Here's the drawing with two shaded views (mm, measured from the low corner). I have some questions. A direction names the side the tool comes from. Round coordinates to 2 decimals unless told otherwise and drop trailing zeros. Order: outer loops, then holes, each group sorted by start corner. A loop starts at its lowest first (then second) coordinate and runs counter-clockwise, first axis right, second up.
Q1. If we section it at A-A (y = 8.5): Please give me the cut outline in (x, z), plus the area to 3 significant figures.
Q2. If we section it at D-D (z = 8): Please give me the cut outline in (x, y), plus the area to 3 significant figures.
Q3. For the marked faces 1 and 2, which set-ups out of +Z, -Z, +X, -X, +Y, -Y let a thin tool reach every point of the face, with its end or its side?
Q4. If I drill on line 1 (Z direction, x = 7.25, y = 3.5); line 2 (Y direction, x = 8.25, z = 32); line 3 (Y direction, x = 12.5, z = 44.5), over which ranges is the centre line in solid material (lowest first)?
Q5. Will these pins go through, and if not, where does the flat tip stop? P1, Ø8, axis at x = 3, z = 16.5, coming from the +Y side; P2, Ø2, axis at x = 14.5, z = 32, coming from the -Y side; P3, Ø2, axis at y = 2, z = 37, coming from the +X side.
Q6. If we section it at C-C (z = 21.5): Please give me the cut outline in (x, y).
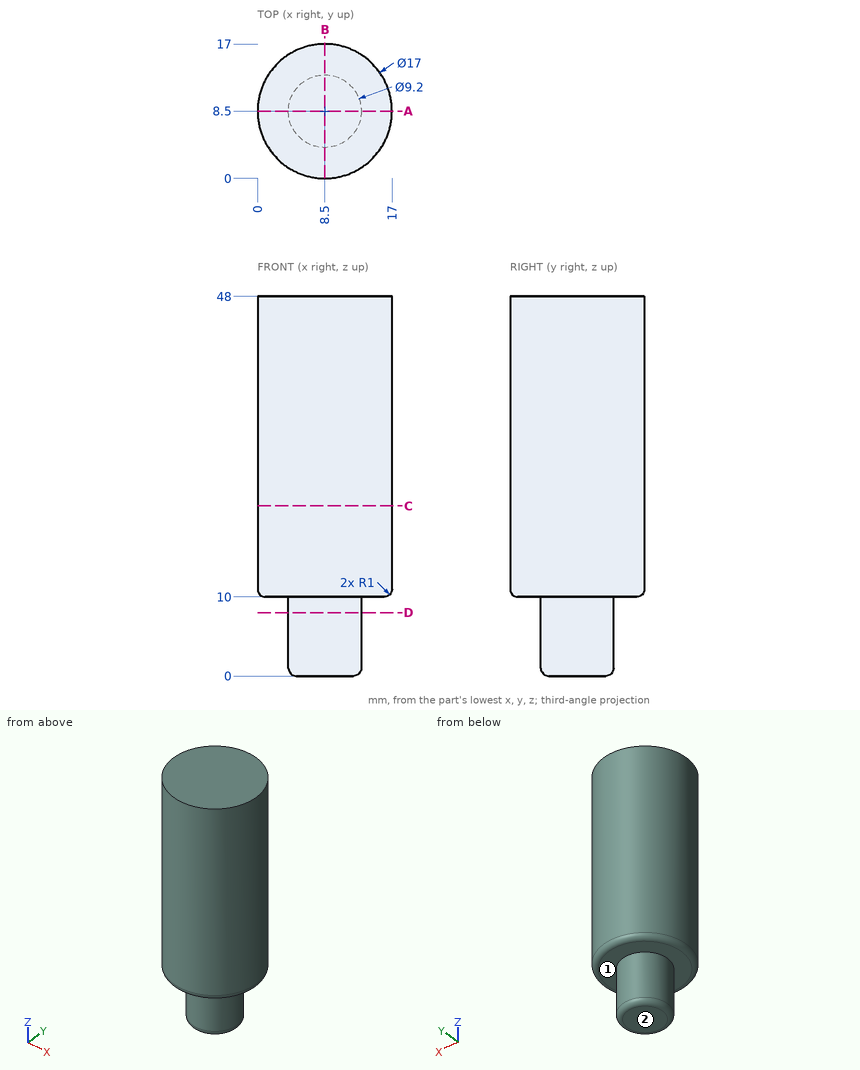
Solution:
1. outline: (0, 11) arc R1 ccw to (1, 10) - (3.9, 10) - (3.9, 1) arc R1 ccw to (4.9, 0) - (12.1, 0) arc R1 ccw to (13.1, 1) - (13.1, 10) - (16, 10) arc R1 ccw to (17, 11) - (17, 48) - (0, 48) - close
1. area: 737 mm2
2. outline: circle Ø9.2 at (8.5, 8.5)
2. area: 66.5 mm2
3. face 1: -Z
3. face 2: -Z, +X, -X, +Y, -Y
4. line 1: z = 10 to 48
4. line 2: y = 0 to 17
4. line 3: y = 1 to 16
5. P1: stops at y = 16.87
5. P2: stops at y = 1.63
5. P3: stops at x = 14.98
6. outline: circle Ø17 at (8.5, 8.5)
